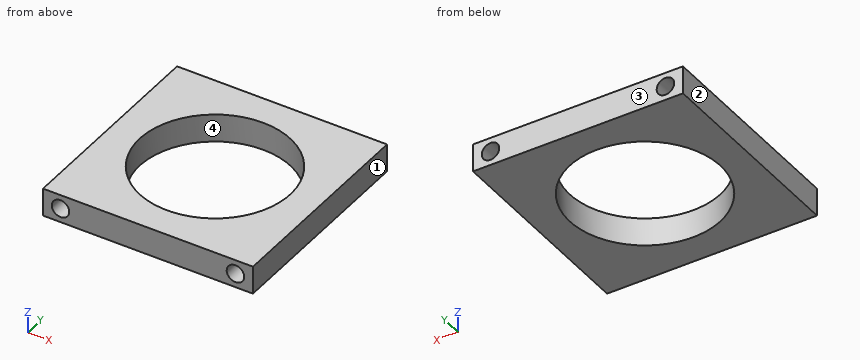
Autodesk Inventor part; units mm, degrees
ref_plane "YZ Plane" through (0, 0, 0) normal (1, 0, 0) x (0, 1, 0)
ref_plane "XZ Plane" through (0, 0, 0) normal (0, 1, 0) x (-1, 0, 0)
ref_plane "XY Plane" through (0, 0, 0) normal (0, 0, 1) x (1, 0, 0)
sketch "Sketch1" plane through (0, 0, 0) normal (0, 0, 1) x (1, 0, 0)
  line L0 (-30, -30) -> (30, -30)
  line L1 (30, -30) -> (30, 30)
  line L2 (30, 30) -> (-30, 30)
  line L3 (-30, 30) -> (-30, -30)
  line L4 (-30, -30) -> (30, 30) construction
  line L5 (30, -30) -> (-30, 30) construction
  point P0 (0, 0)
  dimension "d0" = 60
  dimension "d1" = 60
extrude "Extrusion1" add sketch "Sketch1" along normal blind 8
hole "Hole1" at (0, 0, 0) direction (0, 0, 1) diameter 43 end through all
sketch "Sketch2" plane through (-30, 30, 0) normal (0, 1, 0) x (1, 0, 0)
  line L0 (60, 0) -> (0, 0)
  line L1 (0, 0) -> (0, -8)
  line L2 (60, -8) -> (0, -8)
  line L3 (60, 0) -> (60, -8)
  point P0 (30, 0)
  point P1 (55, -4)
  point P2 (5, -4)
  dimension "d11" = 5
  dimension "d12" = 5
hole "Hole2" at (-25, 30, 4) at (25, 30, 4) direction (0, -1, 0) diameter 5 end through all
properties part number "SpacerSmall"
Can you work these out from the model? Positions are in its coordinate system, mm. Face numbers are marked on the shaded views. Give positions to 0.01 mm unless a question says otherwise; leave off trailing zeros. Loops run counter-clockwise (first coordinate to the right, second up) from the corner with the lowest first, then second, coordinate; pieces in that order, holes last. Notation, with made-up numbers: M 63,65.25 L 117,65.25 A14 ccw 117,80.25 Z; hole C 5,82 d6. An arc over 180 degrees is marked long. Use one line per item in the form item = value. Start each with the question number.
(1) I want a section at D-D, the plane y = 17. Write out the boundary of the cut face in (x, z), and give its area (3 significant figures).
(2) I want a section at B-B, the plane y = 1. Write out the boundary of the cut face in (x, z).
(3) Thinking about a two-plate mould opening in X: for the marked faces 1, 2, 3 and 4, which applies, released by +X, released by -X, zero draft, split by the parting line, or undercut?
(4) I want a section at A-A, the plane z = 4. Write out the boundary of the cut face in (x, y), and give its area (3 significant figures).
(5) Please list where these lines run through material, in increasing order: line 1 (Z direction, x = -25, y = 9); line 2 (Y direction, x = 0, z = 4); line 3 (X direction, y = 22, z = 2.5).
(6) I want a section at C-C, the plane x = 17.5. Write out the boundary of the cut face in (y, z), and give its area (3 significant figures).
(7) I'm going to push a flat-ended pin straight in: P1, Ø5, axis at x = 15, y = -9.5, coming from the +Z side. Where does the tip first touch, or does it pass through?
Worked out:
q1.outline = M -30,0 L -13.16,0 L -13.16,8 L -30,8 Z; M 13.16,0 L 30,0 L 30,8 L 13.16,8 Z; hole C -25,4 d5; hole C 25,4 d5
q1.area = 230 mm²
q2.outline = M -30,0 L -21.48,0 L -21.48,8 L -30,8 Z; M 21.48,0 L 30,0 L 30,8 L 21.48,8 Z; hole C -25,4 d5; hole C 25,4 d5
q3.face_1 = released by +X
q3.face_2 = released by -X
q3.face_3 = zero draft
q3.face_4 = undercut
q4.outline = M -30,-30 L -27.5,-30 L -27.5,30 L -30,30 Z; M -22.5,-30 L 22.5,-30 L 22.5,30 L -22.5,30 Z; M 27.5,-30 L 30,-30 L 30,30 L 27.5,30 Z; hole C 0,0 d43
q4.area = 1,550 mm²
q5.line_1 = 0 to 1.5, 6.5 to 8
q5.line_2 = -30 to -21.5, 21.5 to 30
q5.line_3 = -30 to -27, -23 to 23, 27 to 30
q6.outline = M -30,0 L -12.49,0 L -12.49,8 L -30,8 Z; M 12.49,0 L 30,0 L 30,8 L 12.49,8 Z
q6.area = 280 mm²
q7.P1 = through
